Model file for the job. Use its own axes, mm. A direction names the side the tool comes from. Round coordinates to 2 decimals unless told otherwise and drop trailing zeros. Order: outer loops, then holes, each group sorted by start corner. A loop starts at its lowest first (then second) coordinate and runs counter-clockwise, first axis right, second up. Notation, with made-up numbers: (61, 14) -> (91, 14) arc R13 cw to (91, 31) -> close; hole circle Ø1 at (5.25, 68.25). An arc over 180 degrees is marked (long way). Use CSV: the item, a comma, the result in double quotes.
Autodesk Inventor part; units mm, degrees
ref_plane "YZ Plane" through (0, 0, 0) normal (1, 0, 0) x (0, 1, 0)
ref_plane "XZ Plane" through (0, 0, 0) normal (0, 1, 0) x (-1, 0, 0)
ref_plane "XY Plane" through (0, 0, 0) normal (0, 0, 1) x (1, 0, 0)
sketch "スケッチ1" plane through (0, 0, 0) normal (0, 1, 0) x (-1, 0, 0)
  line L0 (0, 20.7547) -> (0, -42.4528)
  line L1 (68, 12.25) -> (28, 12.25)
  line L2 (28, 12.25) -> (28, 2)
  line L3 (28, 2) -> (0, 2)
  line L4 (68, 12.25) -> (68, 8.25)
  line L5 (68, 8.25) -> (32, 8.25)
  line L6 (32, 8.25) -> (32, 0)
  line L7 (32, 0) -> (0, 0)
  line L8 (-68, 12.25) -> (-28, 12.25)
  line L9 (-28, 12.25) -> (-28, 2)
  line L10 (-28, 2) -> (0, 2)
  line L11 (-68, 12.25) -> (-68, 8.25)
  line L12 (-68, 8.25) -> (-32, 8.25)
  line L13 (-32, 8.25) -> (-32, 0)
  line L14 (-32, 0) -> (0, 0)
  dimension "d0" = 40
  dimension "d1" = 4
  dimension "d2" = 36
  dimension "d3" = 10.25
  dimension "d4" = 2
  dimension "d5" = 56
extrude "押し出し1" add sketch "スケッチ1" along normal blind 20
sketch "スケッチ2" plane through (32, 0, 0) normal (0, 0, -1) x (-1, 0, 0)
  line L0 (0, 0) -> (0, 20)
  line L1 (0, 10) -> (64, 10)
  line L2 (64, 0) -> (64, 20)
  line L3 (32, 0) -> (32, 20)
  line L4 (0, 20) -> (64, 20)
  circle A0 centre (9, 10) radius 1.75
  line L5 (13.1716, 18) -> (13.1716, 2)
  line L6 (13.1716, 2) -> (29.1716, 2)
  line L7 (29.1716, 2) -> (13.1716, 18)
  line L8 (16, 18) -> (32, 18)
  line L9 (16, 18) -> (32, 2)
  circle A1 centre (55, 10) radius 1.75
  line L10 (50.8284, 18) -> (50.8284, 2)
  line L11 (50.8284, 2) -> (34.8284, 2)
  line L12 (34.8284, 2) -> (50.8284, 18)
  line L13 (48, 18) -> (32, 18)
  line L14 (48, 18) -> (32, 2)
  dimension "d8" = 16
  dimension "d9" = 3.5
  dimension "d10" = 2
  dimension "d11" = 46
extrude "押し出し2" cut sketch "スケッチ2" against normal through all contours A0 L1 | L1 A0 | L13 L14 L1 L3 | L3 L1 L9 L8 | L5 L7 L1 | L1 L7 L6 L5 | L3 L9 L1 | L1 L14 L3 | A1 L1 | L1 A1 | L12 L10 L1 | L1 L10 L11 L12
sketch "スケッチ3" plane through (28, 0, 12.25) normal (0, 0, 1) x (1, 0, 0)
  line L0 (-96, 0) -> (-96, 20)
  line L1 (-96, 10) -> (40, 10)
  line L2 (40, 0) -> (40, 20)
  circle A0 centre (27.25, 10) radius 1.75
  circle A1 centre (-83.25, 10) radius 1.75
  point P0 (-28, 0)
  dimension "d14" = 3.5
  dimension "d15" = 12.75
  dimension "d16" = 12.75
extrude "押し出し3" cut sketch "スケッチ3" against normal through all
fillet "フィレット1" radius 2 4 edges at (-68, 20, 10.25) (68, 20, 10.25) (68, 0, 10.25) (-68, 0, 10.25)
fillet "フィレット2" radius 2 4 edges at (-28, 10, 2) (-28, 10, 12.25) (28, 10, 2) (28, 10, 12.25)
properties part number "axis3"
Q1. Cut at D-D (x = 39). Give the cut face in (y, z), plus the area to 3 significant figures.
From the geometry:
outline,"(0, 8.25) -> (20, 8.25) -> (20, 12.25) -> (0, 12.25) -> close"
area,"80.0 mm²"
Q2. Cut at A-A (x = 23). Give the cut face in (y, z).
From the geometry:
outline,"(0, 0) -> (8.25, 0) -> (8.25, 2) -> (0, 2) -> close; (11.75, 0) -> (20, 0) -> (20, 2) -> (11.75, 2) -> close"
Q3. Probe line 1 along X through (y, z) = (10.25, 10.5); line 2 along X through (y, z) = (16, 4.5); line 3 along Y through (x, z) = (55.25, 9.95). List the from-to ranges inside material, lowest first.
From the geometry:
line 1,"x = -68 to -56.98, -53.52 to -28.02, 28.02 to 53.52, 56.98 to 68"
line 2,"x = -32 to -28, 28 to 32"
line 3,"y = 0 to 8.25, 11.75 to 20"
Q4. Pin check, flat tips, straight feed: pin 1 (2.5 mm diameter, centred on y = 14, z = 5.5, fed in from -X); pin 2 (5.5 mm diameter, centred on x = -55.25, y = 10, fed in from -Z); pin 3 (3 mm diameter, centred on x = 20.5, y = 12.5, fed in from +Z). Stop position of each tip, or through.
From the geometry:
pin 1,"stops at x = -32"
pin 2,"stops at z = 8.25"
pin 3,"stops at z = 2"
Q5. Cut at B-B (z = 7). Give the cut face in (x, y), plus the area to 3 significant figures.
From the geometry:
outline,"(-32, 0) -> (-28, 0) -> (-28, 20) -> (-32, 20) -> close; (28, 0) -> (32, 0) -> (32, 20) -> (28, 20) -> close"
area,"160 mm²"
Q6. Cut at C-C (y = 6.25). Give the cut face in (x, z).
From the geometry:
outline,"(-68, 8.25) -> (-32, 8.25) -> (-32, 0) -> (-18.83, 0) -> (-18.83, 2) -> (-26, 2) arc R2 cw to (-28, 4) -> (-28, 10.25) arc R2 ccw to (-30, 12.25) -> (-68, 12.25) -> close; (-7.08, 0) -> (-4.25, 0) -> (-4.25, 2) -> (-7.08, 2) -> close; (4.25, 0) -> (7.08, 0) -> (7.08, 2) -> (4.25, 2) -> close; (18.83, 0) -> (32, 0) -> (32, 8.25) -> (68, 8.25) -> (68, 12.25) -> (30, 12.25) arc R2 ccw to (28, 10.25) -> (28, 4) arc R2 cw to (26, 2) -> (18.83, 2) -> close"
Q7. Mould opens along X. For faces 4 (the cylindrical face through (-21.25, 10.08, 0.99)), 5 (the flat face through (68, 10, 10)), 6 (the flat face through (49, 10, 12.25)), 7 (the flat face through (-32, 10, 4)) say: +X half, -X half, draft (parallel to the pull), parting line (faces both ways), or undercut.
From the geometry:
face 4,"undercut"
face 5,"+X half"
face 6,"draft"
face 7,"-X half"
Q8. Which spindle directions (+Z, -Z, +X, -X, +Y, -Y) get a long thin tool onto all of the face, cutting with end or side? Do faces 1 (the flat face through (8, 10, 1)), 2 (the flat face through (28, 10, 7)), 3 (the flat face through (50, 10, 8.25)). Say none if no direction does.
From the geometry:
face 1,"+Z, -Z"
face 2,"+Z, +Y, -Y"
face 3,"-Z, +X, +Y, -Y"
